Here's how the part is built. I have some questions about the finished solid (model axes, mm). A direction names the side the tool comes from. Give positions to 0.01 mm unless a question says otherwise; leave off trailing zeros. Write each loop counter-clockwise with the first axis right and the second up, starting at its lowest first coordinate (ties: lowest second). Pieces come first, ordered by that corner, then holes. Notation, with made-up numbers: (58.25, 44) - (91.25, 44) arc R29 cw to (91.25, 65) - close; hole circle Ø9 at (16, -25). An arc over 180 degrees is marked (long way). Use a Markdown table: item, result.
Autodesk Inventor part; units mm, degrees
ref_plane "WorkPlane1" through (0, 0, 0) normal (0, 0, 1) x (1, 0, 0)
ref_plane "MSC_PF1" through (0, 0, 0) normal (1, 0, 0) x (0, 1, 0)
ref_plane "MSC_PT1" through (0, 0, 0) normal (0, 0, -1) x (-1, 0, 0)
ref_plane "WorkPlane1" through (0, 0, 0) normal (0, 0, 1) x (1, 0, 0)
sketch "Sketch1" plane through (0, 0, 0) normal (0, 0, 1) x (1, 0, 0)
  point P0 (0, 0)
sketch "Sketch2" plane through (0, 0, 0) normal (0, 0, 1) x (1, 0, 0)
  line L0 (-18, 10.3926) -> (-18, -10.3926)
  line L1 (0, 20.7843) -> (-18, 10.3926)
  line L2 (18, 10.3926) -> (0, 20.7843)
  line L3 (18, -10.3926) -> (18, 10.3926)
  line L4 (0, -20.7843) -> (18, -10.3926)
  line L5 (-18, -10.3926) -> (0, -20.7843)
  circle A0 centre (0, 0) radius 18 construction
  dimension "d1" = 36
  dimension "d29" = 0
  dimension "d30" = 0
extrude "Extrusion1" add sketch "Sketch2" along normal blind 15
sketch "Sketch3" plane through (0, 0, 0) normal (1, 0, 0) x (0, 1, 0)
  line L0 (18, 15) -> (20.8843, 15)
  line L1 (20.8843, 13.3347) -> (18, 15)
  line L2 (20.8843, 15) -> (20.8843, 13.3347)
  line L3 (0, -3) -> (0, 18)
  line L4 (20.7843, 0) -> (20.7843, 15)
  dimension "d25" = 0.1
  dimension "d26" = 0
  dimension "d27" = 60
  dimension "d28" = 18
revolve "Revolution1" cut sketch "Sketch3" angle 360 about axis through (0, 0, -10) along (0, 0, 1)
sketch "Sketch4" plane through (0, 0, 0) normal (1, 0, 0) x (0, 1, 0)
  line L0 (0, -100) -> (0, 0)
  line L1 (-12, -100) -> (0, -100)
  line L2 (-12, 0) -> (-12, -100)
  line L3 (0, 0) -> (-12, 0)
  line L4 (0, -100) -> (0, 0)
  line L5 (-14.4, 0) -> (2.4, 0)
  line L6 (0, -120) -> (0, 20)
  dimension "d18" = 12
  dimension "d20" = 100
  dimension "d33" = 0
  dimension "d34" = 0
revolve "Revolution2" add sketch "Sketch4" angle 360 about axis through (0, 0, -100) along (0, 0, -1)
chamfer "Chamfer1" distance 1.5 angle 45 1 edges at (0, 12, -100)
fillet "Fillet1" radius 0.8 1 edges at (0, 12, 0)
thread "Thread1"
ref_plane "MSC_PF1" through (0, 0, 0) normal (1, 0, 0) x (0, 1, 0)
ref_plane "MSC_PT1" through (0, 0, 0) normal (0, 0, -1) x (-1, 0, 0)
equation "\"d22\" = 0.5 * PTC"
equation "\"d23\" = 0.5 * PTC"
equation "\"d24\" = r"
equation "\"d1\" = ParS"
equation "\"d6\" = ParK"
equation "\"d28\" = 0.5 * ParS"
equation "\"d18\" = 0.5 * NND"
equation "\"d20\" = NLG"
equation "\"NND\" = 24"
equation "\"NLG\" = 100"
equation "\"PTC\" = 3"
equation "\"ParK\" = 15"
equation "\"ParS\" = 36"
equation "\"msp_es\" = 0.577367 * ParS"
equation "\"r\" = 0.8"
equation "\"THREADDIA\" = NND"
properties part number "ISO 4016 - M24 x 100" material "Steel"
Item 1: I need wall thicknesses on line 1 along Z through (x, y) = (4, 13.5); line 2 along Y through (x, z) = (9.5, -48.5); line 3 along X through (y, z) = (9, -27). Which ranges of each line are inside material? Lowest first, please. Write a range as [from, to].
Values:
| item | result |
|---|---|
| line 1 | z = [0, 15] |
| line 2 | y = [-7.33, 7.33] |
| line 3 | x = [-7.94, 7.94] |
Item 2: For faces 1 (the conical face through (16.197, -9.299, 14.609)), 2 (the cylindrical face through (-0.53, 11.99, -50.33)), which set-ups out of +Z, -Z, +X, -X, +Y, -Y let a thin tool reach every point of the face, with its end or its side?
Values:
| item | result |
|---|---|
| face 1 | +Z, +X, -Y |
| face 2 | -Z |
Item 3: Will these pins go through, and if not, where does the flat tip stop? pin 1 Ø5 at (y, z) = (15.5, -37) entering from -X; pin 2 Ø5 at (y, z) = (-0.5, -85) entering from -X; pin 3 Ø12 at (x, z) = (-6.5, -4) entering from +Y; pin 4 Ø3 at (x, y) = (10, 15.5) entering from +Z.
Values:
| item | result |
|---|---|
| pin 1 | passes through |
| pin 2 | stops at x = -12 |
| pin 3 | stops at y = 19.61 |
| pin 4 | stops at z = 15 |
Item 4: If we section it at A-A, the plane z = -85: Write out the boundary of the cut face in (x, y), plus the area to 3 significant figures.
Values:
| item | result |
|---|---|
| outline | circle Ø24 at (0, 0) |
| area | 452 mm2 |
